Verification items for the finished model (mm, model axes). Face numbers are marked on the shaded views. A direction names the side the tool comes from. Coordinates: 2 decimals unless noted, no trailing zeros. Write each loop counter-clockwise with the first axis right and the second up, starting at its lowest first coordinate (ties: lowest second). Pieces come first, ordered by that corner, then holes. Notation, with made-up numbers: (-7, -3) -> (42, -3) arc R16 cw to (42, 2) -> close; hole circle Ø11 at (-11.5, -15.75). An arc over 180 degrees is marked (long way). Answer in a Markdown table with one row per item.
```python
from build123d import *

# Parameters (mm, degrees)
SKETCH1_W           = 40
SKETCH1_H           = 30
BOSS_EXTRUDE1_DEPTH = 10
SKETCH2_R           = 1.55
SKETCH2_R_2         = 6.25
CUT_EXTRUDE1_DEPTH  = 4
SKETCH3_R           = 4.8125
CUT_EXTRUDE2_DEPTH  = 10


with BuildPart() as part:
    # Sketch1 → Boss-Extrude1 (new body)
    with BuildSketch(Plane(origin=(0, 0, 0), x_dir=(1, 0, 0), z_dir=(0, 1, 0))):
        Rectangle(SKETCH1_W, SKETCH1_H)
    extrude(amount=BOSS_EXTRUDE1_DEPTH)

    # Sketch2 → Cut-Extrude1 (cut)
    with BuildSketch(Plane(origin=(0, 0, 0), x_dir=(-1, 0, 0), z_dir=(0, -1, 0))):
        with Locations(Location((13.333333333, -10, 0), (0, 0, 90))):
            Circle(SKETCH2_R)
        with Locations(Location((13.333333333, 10, 0), (0, 0, 270))):
            Circle(SKETCH2_R)
        with Locations(Location((-13.333333333, 10, 0), (0, 0, 90))):
            Circle(SKETCH2_R)
        with Locations(Location((-8.14, -6.75, 0), (0, 0, 90))):
            Circle(SKETCH2_R_2)
    extrude(amount=-CUT_EXTRUDE1_DEPTH, mode=Mode.SUBTRACT)

    # Sketch3 → Cut-Extrude2 (cut)
    with BuildSketch(Plane(origin=(0, 10, 0), x_dir=(1, 0, 0), z_dir=(0, 1, 0))):
        with Locations(Location((8.14, -6.75, 0), (0, 0, 270))):
            Circle(SKETCH3_R)
    extrude(amount=-CUT_EXTRUDE2_DEPTH, mode=Mode.SUBTRACT)


solid = part.part
```
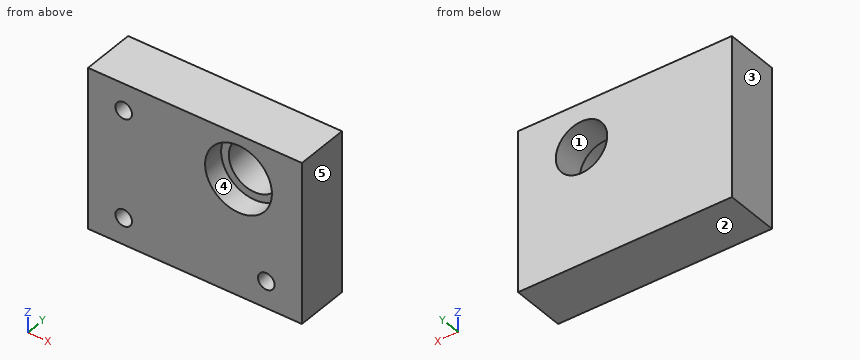
1. Thickness scan on line 1 (X direction, y = 3.05, z = -10); line 2 (X direction, y = 6, z = 6.75); line 3 (X direction, y = 2, z = 10). Record the ranges inside material, lowest first. Write a range as from..to.
Geometry says:
| item | result |
|---|---|
| line 1 | -20..-14.88, -11.78..11.78, 14.88..20 |
| line 2 | -20..3.33, 12.95..20 |
| line 3 | -20..-14.88, -11.78..2.8, 13.48..20 |
2. Depth check by flat-ended pin: P1, Ø1.6, axis at x = -13, z = 10.5, coming from the -Y side. Enter the tip coordinate at first touch or a pass-through.
Geometry says:
| item | result |
|---|---|
| P1 | y = 4 |
3. Section check A-A, the plane x = 8.14. Record the boundary of the cut face in (y, z), plus the area to 3 significant figures.
Geometry says:
| item | result |
|---|---|
| outline | (0, -15) -> (10, -15) -> (10, 1.94) -> (4, 1.94) -> (4, 0.5) -> (0, 0.5) -> close; (0, 13) -> (4, 13) -> (4, 11.56) -> (10, 11.56) -> (10, 15) -> (0, 15) -> close |
| area | 192 mm^2 |
4. Tool access check on the marked faces 4 and 5. Record the directions out of +Z, -Z, +X, -X, +Y, -Y that give a thin tool (end or side, any length) a straight path to the whole face; none if there is none.
Geometry says:
| item | result |
|---|---|
| face 4 | -Y |
| face 5 | +Z, -Z, +X, +Y, -Y |
5. Mould release check, pull along X, two halves, no side actions. Record for the marked faces 1, 2 and 3: released by +X, released by -X, zero draft, split by the parting line, or undercut.
Geometry says:
| item | result |
|---|---|
| face 1 | undercut |
| face 2 | zero draft |
| face 3 | released by -X |
6. Section check D-D, the plane z = -10. Record the boundary of the cut face in (x, y).
Geometry says:
| item | result |
|---|---|
| outline | (-20, 0) -> (-14.88, 0) -> (-14.88, 4) -> (-11.78, 4) -> (-11.78, 0) -> (11.78, 0) -> (11.78, 4) -> (14.88, 4) -> (14.88, 0) -> (20, 0) -> (20, 10) -> (-20, 10) -> close |
7. Section check B-B, the plane z = 6.75. Record the boundary of the cut face in (x, y).
Geometry says:
| item | result |
|---|---|
| outline | (-20, 0) -> (1.89, 0) -> (1.89, 4) -> (3.33, 4) -> (3.33, 10) -> (-20, 10) -> close; (12.95, 4) -> (14.39, 4) -> (14.39, 0) -> (20, 0) -> (20, 10) -> (12.95, 10) -> close |
